Read the model definition and answer for the solid it produces. Units are mm, in the model's axes. Face numbers are marked on the shaded views. A direction names the side the tool comes from. Round coordinates to 2 decimals unless told otherwise and drop trailing zeros. Loops run counter-clockwise (first coordinate to the right, second up) from the corner with the lowest first, then second, coordinate; pieces in that order, holes last. Notation, with made-up numbers: (-39, 43) - (8, 43) arc R27 cw to (8, 65) - close; hole circle Ø2 at (36.5, -15). An arc over 180 degrees is marked (long way). Answer as CSV lines item,"result".
```python
from build123d import *

# Parameters (mm, degrees)
F0_R     = 17
F1_DEPTH = 3
F3_DEPTH = 10
F4_R     = 10
F5_DEPTH = 10
F6_R     = 10
F7_DEPTH = 10
F8_R     = 8.75
F9_DEPTH = 13.001


with BuildPart() as f1:
    # F0 (on Top) → F1 (new body)
    with BuildSketch(Plane.XY):
        Circle(F0_R)
    extrude(amount=F1_DEPTH)

    # F2 (on face) → F3 (join)
    with BuildSketch(Plane.XY.offset(3)):
        Polygon((-12, 16), (-30, 16), (-30, -14), (-12, -14), (12, -14), (30, -14), (30, 16), (12, 16), align=None)
        with BuildLine():
            ThreePointArc((12, 16), (0, 20), (-12, 16))
            Line((-12, 16), (12, 16))
        make_face()
        with BuildLine():
            Line((12, -14), (-12, -14))
            ThreePointArc((-12, -14), (0, -18.4390889146), (12, -14))
        make_face()
    extrude(amount=F3_DEPTH)

    # F4 (on face) → F5 (join)
    with BuildSketch(Plane.YZ.offset(30)):
        with BuildLine():
            Line((-14, 35), (-14, 13))
            Line((-14, 13), (16, 13))
            Line((16, 13), (16, 35))
            ThreePointArc((16, 35), (1, 50), (-14, 35))
        make_face()
        with Locations((1, 35)):
            Circle(F4_R, mode=Mode.SUBTRACT)
    extrude(amount=-F5_DEPTH)

    # F6 (on face) → F7 (join)
    with BuildSketch(Plane(origin=(-30, 0, 0), x_dir=(0, -1, 0), z_dir=(-1, 0, 0))):
        with BuildLine():
            Line((-16, 35), (-16, 13))
            Line((-16, 13), (14, 13))
            Line((14, 13), (14, 35))
            ThreePointArc((14, 35), (-1, 50), (-16, 35))
        make_face()
        with Locations((-1, 35)):
            Circle(F6_R, mode=Mode.SUBTRACT)
    extrude(amount=-F7_DEPTH)

    # F8 (on face) → F9 (cut, through all)
    with BuildSketch(Plane.XY.offset(13)):
        Circle(F8_R)
    extrude(amount=-F9_DEPTH, mode=Mode.SUBTRACT)


solid = f1.part
```
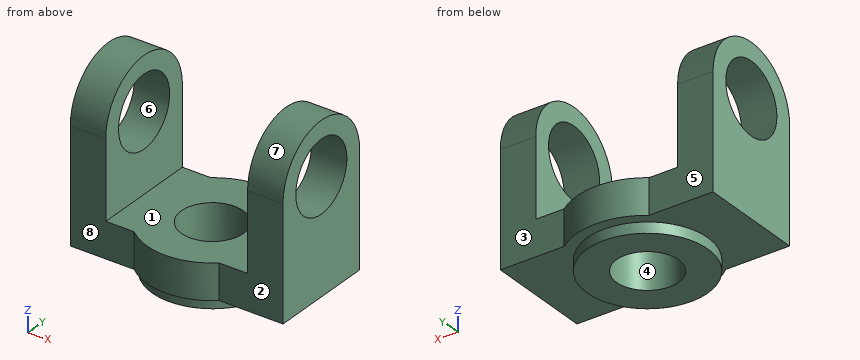
1) A cutting plane is placed at A-A, the plane z = 4. Determine the outline of the cut face in (x, y), plus the area to 3 significant figures.
Entries:
outline,"(-30, -14) - (-12, -14) arc R18.44 ccw to (12, -14) - (30, -14) - (30, 16) - (12, 16) arc R20 ccw to (-12, 16) - (-30, 16) - close; hole circle Ø17.5 at (0, 0)"
area,"1,700 mm^2"
2) The mould has two halves that part along Z. Classify the marked faces 6, 7 and 8: pulls with the +Z half, pulls with the -Z half, needs draft (parallel to the pull), parting line crosses it, or undercut.
Entries:
face 6,"undercut"
face 7,"pulls with the +Z half"
face 8,"needs draft"
3) Each of these flat-tipped pins is pushed along its axis until it touches: P1, Ø5, axis at x = 24, z = 24, coming from the +Y side; P2, Ø11.5, axis at x = 6, y = -0.5, coming from the +Z side; P3, Ø6, axis at x = 24, y = -6.5, coming from the -Z side; P4, Ø14, axis at x = 0, y = 0, coming from the +Z side. Where does it stop, or does it pass through?
Entries:
P1,"stops at y = 16"
P2,"stops at z = 13"
P3,"stops at z = 3"
P4,"passes through"
4) A cutting plane is placed at B-B, the plane x = 0. Determine the outline of the cut face in (y, z).
Entries:
outline,"(-18.44, 3) - (-17, 3) - (-17, 0) - (-8.75, 0) - (-8.75, 13) - (-18.44, 13) - close; (8.75, 0) - (17, 0) - (17, 3) - (20, 3) - (20, 13) - (8.75, 13) - close"
5) Find the intervals of material crossed by line 1 (Y direction, x = 0, z = 5); line 2 (X direction, y = -6, z = 44.5); line 3 (Z direction, x = 28, y = 1), in increasing order.
Entries:
line 1,"y = -18.44 to -8.75, 8.75 to 20"
line 2,"x = -30 to -20, 20 to 30"
line 3,"z = 3 to 25, 45 to 50"
6) A cutting plane is placed at C-C, the plane z = 14. Determine the outline of the cut face in (x, y), plus the area to 3 significant figures.
Entries:
outline,"(-30, -14) - (-20, -14) - (-20, 16) - (-30, 16) - close; (20, -14) - (30, -14) - (30, 16) - (20, 16) - close"
area,"600 mm^2"
7) A cutting plane is placed at D-D, the plane y = 0. Determine the outline of the cut face in (x, z).
Entries:
outline,"(-30, 3) - (-17, 3) - (-17, 0) - (-8.75, 0) - (-8.75, 13) - (-20, 13) - (-20, 25.05) - (-30, 25.05) - close; (-30, 44.95) - (-20, 44.95) - (-20, 49.97) - (-30, 49.97) - close; (8.75, 0) - (17, 0) - (17, 3) - (30, 3) - (30, 25.05) - (20, 25.05) - (20, 13) - (8.75, 13) - close; (20, 44.95) - (30, 44.95) - (30, 49.97) - (20, 49.97) - close"
8) A tool of negligible diameter and unlimited length cuts with its end or side. For the marked faces 1, 2, 3, 4 and 5, from which of +Z, -Z, +X, -X, +Y, -Y can it reach the whole face along a straight path? Write none if from no direction.
Entries:
face 1,"+Z, +Y, -Y"
face 2,"+Z, -Z, +X, -Y"
face 3,"+Z, -Z, +X, +Y"
face 4,"+Z, -Z"
face 5,"+Z, -Z, -X, +Y"
